Check sheet for the modelled part. Datum: model origin and axes. Units: mm. A direction names the side the tool comes from. Round coordinates to 2 decimals unless told otherwise and drop trailing zeros. Order: outer loops, then holes, each group sorted by start corner. A loop starts at its lowest first (then second) coordinate and runs counter-clockwise, first axis right, second up. Notation, with made-up numbers: M -14.5,17 L 22.5,17 A32 cw 22.5,49 Z; hole C 19.25,47 d9. An arc over 180 degrees is marked long. One line per item, written item: value. Start each with the question number.
(1) Depth check by flat-ended pin: pin 1 Ø1.5 at (x, z) = (20, -2) entering from -Y; pin 2 Ø1 at (x, z) = (66, -1.5) entering from +Y; pin 3 Ø0.6 at (x, z) = (99, 1) entering from -Y. Enter the tip coordinate at first touch or a pass-through.
(2) Cross-section at B-B, the plane x = 17. Enter the section's corners in (y, z).
(3) Release check for a two-part mould opening along Y. For faces 6 (the face through (100, -2, 0)), 7 (the face through (99.8, 4.2, 0.1)), 8 (the face through (99, -0.75, 0)) record: released by +Y, released by -Y, zero draft, split by the parting line, or undercut.
(4) Access from +Z, -Z, +X, -X, +Y, -Y to the whole of each face (thin tool, end or side, straight path). Record for faces 1 (the face through (53.64, -1.08, -4.88)), 2 (the face through (99, 0.75, 0)), 3 (the face through (6.507, 3.233, -1.341)), 4 (the face through (0, 0, 0)), 5 (the face through (3.535, -0.867, -3.905)).
(5) Thickness scan on L1, parallel to X at y = 3.75, z = -0.5; L2, parallel to X at y = 0.5, z = -4; L3, parallel to Z at x = 96, y = 0.25. Record the ranges inside material, lowest first.
(6) Cross-section at A-A, the plane z = 0. Enter the section's corners in (x, y), and give its area (3 significant figures).
Autodesk Inventor part; units mm, degrees
ref_plane "YZ Plane" through (0, 0, 0) normal (1, 0, 0) x (0, 1, 0)
ref_plane "XZ Plane" through (0, 0, 0) normal (0, 1, 0) x (-1, 0, 0)
ref_plane "XY Plane" through (0, 0, 0) normal (0, 0, 1) x (1, 0, 0)
sketch "Sketch1" plane through (0, 0, 0) normal (0, 0, 1) x (1, 0, 0)
  line L0 (0, 0) -> (0, 4)
  line L1 (0, 4) -> (6, 4)
  line L2 (7, 3.5) -> (7, 5)
  line L3 (7, 5) -> (100, 5)
  line L4 (100, 5) -> (100, 0)
  line L5 (100, 0) -> (0, 0)
  line L6 (6, 4) -> (6, 3.5)
  line L7 (6, 3.5) -> (7, 3.5)
  dimension "d0" = 8
  dimension "d1" = 10
  dimension "d3" = 100
  dimension "d17" = 7
  dimension "d18" = 1
  dimension "d19" = 7
revolve "Revolution1" add sketch "Sketch1" angle 360 about axis through (100, 0, 0) along (-1, 0, 0)
thread "Thread1"
chamfer "Chamfer1" distance 1 angle 45 1 edges at (0, -4, 0)
sketch "Sketch2" plane through (0, 0, 0) normal (0, 0, 1) x (1, 0, 0)
  line L0 (100, 0.75) -> (98, 0.75)
  line L1 (98, 0.75) -> (98, -0.75)
  line L2 (98, -0.75) -> (100, -0.75)
  line L3 (100, -0.75) -> (100, 0.75)
  line L4 (100, -5) -> (100, 5) construction
  point P0 (0, 0)
  point P1 (98, 0)
  dimension "d10" = 1.5
  dimension "d11" = 2
extrude "Extrusion1" cut sketch "Sketch2" along normal through all both and the other way through all
chamfer "Chamfer2" distance 1 angle 45 3 edges at (100, -5, 0) (100, 3.7914, -3.2596) (100, 3.7914, 3.2596)
properties part number "Shaft" material "Steel"
Values found:
1. pin 1: y = -4.84
1. pin 2: y = 4.9
1. pin 3: y = -4.95
2. outline: C 0,0 d10
3. face 6: zero draft
3. face 7: released by +Y
3. face 8: undercut
4. face 1: +X, -X
4. face 2: +Z, -Z, +X
4. face 3: none
4. face 4: +Z, -Z, -X, +Y, -Y
4. face 5: -X
5. L1: 0.78 to 6, 7 to 100
5. L2: 7 to 98
5. L3: -4.99 to 4.99
6. outline: M 0,-3 L 1,-4 L 6,-4 L 6,-3.5 L 7,-3.5 L 7,-5 L 99,-5 L 100,-4 L 100,-0.75 L 98,-0.75 L 98,0.75 L 100,0.75 L 100,4 L 99,5 L 7,5 L 7,3.5 L 6,3.5 L 6,4 L 1,4 L 0,3 Z
6. area: 980 mm^2
